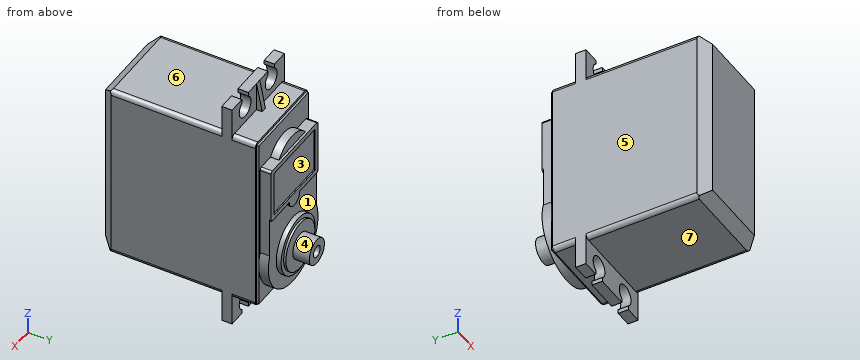
from build123d import *

# Parameters (mm, degrees)
SKETCH1_W           = 20
SKETCH1_H           = 40.5
BOSS_EXTRUDE1_DEPTH = 35.2
CHAMFER1_SIZE       = 2
CHAMFER1_SIZE2      = 2.383507185
BOSS_EXTRUDE2_DEPTH = 2.3
SKETCH3_W           = 1.25
SKETCH3_H           = 6.5
BOSS_EXTRUDE3_DEPTH = 1.3
CHAMFER2_SIZE       = 6.687920221
CHAMFER2_SIZE_2     = 1.3
SKETCH5_OUTSIDE_W   = 35.418
SKETCH5_OUTSIDE_H   = 68.918
SKETCH5_OUTSIDE_W_2 = 19
SKETCH5_OUTSIDE_H_2 = 39.5
CUT_EXTRUDE1_DEPTH  = 0.5
BOSS_EXTRUDE4_DEPTH = 2.15
BOSS_EXTRUDE5_DEPTH = 1.9
SKETCH8_R           = 6.5
BOSS_EXTRUDE6_DEPTH = 1.1
SKETCH9_R           = 5.55
BOSS_EXTRUDE7_DEPTH = 0.5
SKETCH10_R          = 2.9
SKETCH10_R_2        = 1.3
BOSS_EXTRUDE8_DEPTH = 3.7
SKETCH11_W          = 15.8
SKETCH11_H          = 10.3
BOSS_EXTRUDE9_DEPTH = 0.3
FILLET1_R           = 0.5
FILLET2_R           = 1


with BuildPart() as part:
    # Sketch1 → Boss-Extrude1 (new body)
    with BuildSketch(Plane(origin=(0, 0, 0), x_dir=(1, 0, 0), z_dir=(0, 1, 0))):
        with Locations((0, -10.25)):
            Rectangle(SKETCH1_W, SKETCH1_H)
    extrude(amount=BOSS_EXTRUDE1_DEPTH)

    # Chamfer1
    chamfer1_edges = [part.edges().sort_by_distance(p)[0] for p in [
        (0, 0, 30.5),
        (-10, 0, 10.25),
        (0, 0, -10),
        (10, 0, 10.25),
    ]]
    chamfer1_side = [part.faces().sort_by_distance(p)[0] for p in [
        (0, 0, 10.25),
    ]]
    chamfer(chamfer1_edges, length=CHAMFER1_SIZE, length2=CHAMFER1_SIZE2, reference=chamfer1_side[0])

    # Sketch2 → Boss-Extrude2 (add)
    with BuildSketch(Plane(origin=(0, 27.2, 0), x_dir=(-1, 0, 0), z_dir=(0, 1, 0))):
        with BuildLine():
            Line((10, -10), (-10, -10))
            Line((-10, -10), (-10, -16.5))
            Line((-10, -16.5), (-6.25, -16.5))
            Line((-6.25, -16.5), (-6.25, -15.570828693))
            ThreePointArc((-6.25, -15.570828693), (-5, -11.45), (-3.75, -15.570828693))
            Line((-3.75, -15.570828693), (-3.75, -16.5))
            Line((-3.75, -16.5), (3.75, -16.5))
            Line((3.75, -16.5), (3.75, -15.570828693))
            ThreePointArc((3.75, -15.570828693), (5, -11.45), (6.25, -15.570828693))
            Line((6.25, -15.570828693), (6.25, -16.5))
            Line((6.25, -16.5), (10, -16.5))
            Line((10, -16.5), (10, -10))
        make_face()
        with BuildLine():
            Line((-6.25, 37), (-10, 37))
            Line((-10, 37), (-10, 30.5))
            Line((-10, 30.5), (10, 30.5))
            Line((10, 30.5), (10, 37))
            Line((10, 37), (6.25, 37))
            Line((6.25, 37), (6.25, 36.070828693))
            ThreePointArc((6.25, 36.070828693), (5, 31.95), (3.75, 36.070828693))
            Line((3.75, 36.070828693), (3.75, 37))
            Line((3.75, 37), (-3.75, 37))
            Line((-3.75, 37), (-3.75, 36.070828693))
            ThreePointArc((-3.75, 36.070828693), (-5, 31.95), (-6.25, 36.070828693))
            Line((-6.25, 36.070828693), (-6.25, 37))
        make_face()
    extrude(amount=BOSS_EXTRUDE2_DEPTH)

    # Sketch3 → Boss-Extrude3 (add)
    with BuildSketch(Plane(origin=(0, 29.5, 0), x_dir=(1, 0, 0), z_dir=(0, 1, 0))):
        with Locations((0, -33.75)):
            Rectangle(SKETCH3_W, SKETCH3_H)
        with Locations((0, 13.25)):
            Rectangle(SKETCH3_W, SKETCH3_H)
    extrude(amount=BOSS_EXTRUDE3_DEPTH)

    # Chamfer2
    # the kernel refuses this chamfer: 6.687920221, 1.3 mm, written as the material it takes off along each edge
    with BuildSketch(Plane(origin=(-18.001773564, 30.8, 37), x_dir=(0, 0.007343799087842576, -0.9999730339438946), z_dir=(1, 0, 0))) as chamfer2_piece_1_section:
        Polygon((CHAMFER2_SIZE * 0.999973033908, -CHAMFER2_SIZE * 0.00734379908758), (-CHAMFER2_SIZE_2 * 0.00734379908784, -CHAMFER2_SIZE_2 * 0.999973033944), (0, 0), align=None)
    chamfer2_piece_1 = extrude(amount=36.003547128, mode=Mode.PRIVATE)
    chamfer2_piece_1 = split(chamfer2_piece_1, bisect_by=Plane(origin=(0, 30.433956973, 30.5), z_dir=(0, 0, 1)), keep=Keep.TOP, mode=Mode.PRIVATE)
    add(chamfer2_piece_1, mode=Mode.SUBTRACT)
    with BuildSketch(Plane(origin=(18.001773564, 30.8, -16.5), x_dir=(0, -0.9816291836389949, -0.19079870499623547), z_dir=(-1, 0, 0))) as chamfer2_piece_2_section:
        Polygon((CHAMFER2_SIZE_2 * 0.981629183639, CHAMFER2_SIZE_2 * 0.190798704996), (-CHAMFER2_SIZE * 0.190798704989, CHAMFER2_SIZE * 0.981629183604), (0, 0), align=None)
    chamfer2_piece_2 = extrude(amount=36.003547128, mode=Mode.PRIVATE)
    chamfer2_piece_2 = split(chamfer2_piece_2, bisect_by=Plane(origin=(0, 30.433956973, -10), z_dir=(0, 0, -1)), keep=Keep.TOP, mode=Mode.PRIVATE)
    add(chamfer2_piece_2, mode=Mode.SUBTRACT)

    # Sketch5 outside → Cut-Extrude1 (cut)
    with BuildSketch(Plane(origin=(0, 35.2, 0), x_dir=(1, 0, 0), z_dir=(0, 1, 0))):
        with Locations((0, -10.25)):
            Rectangle(SKETCH5_OUTSIDE_W, SKETCH5_OUTSIDE_H)
        with Locations((0, -10.25)):
            Rectangle(SKETCH5_OUTSIDE_W_2, SKETCH5_OUTSIDE_H_2, mode=Mode.SUBTRACT)
    extrude(amount=-CUT_EXTRUDE1_DEPTH, mode=Mode.SUBTRACT)

    # Sketch6 → Boss-Extrude4 (add)
    with BuildSketch(Plane(origin=(0, 35.2, 0), x_dir=(1, 0, 0), z_dir=(0, 1, 0))):
        with BuildLine():
            Line((-9, -3.041381265), (-9, -24.1))
            Line((-9, -24.1), (9, -24.1))
            Line((9, -24.1), (9, -3.041381265))
            ThreePointArc((9, -3.041381265), (0, 9.5), (-9, -3.041381265))
        make_face()
    extrude(amount=BOSS_EXTRUDE4_DEPTH)

    # Sketch7 → Boss-Extrude5 (add)
    with BuildSketch(Plane(origin=(0, 35.2, 0), x_dir=(1, 0, 0), z_dir=(0, 1, 0))):
        with BuildLine():
            Line((-5, -24.1), (5, -24.1))
            ThreePointArc((5, -24.1), (0, -26.6), (-5, -24.1))
        make_face()
    extrude(amount=BOSS_EXTRUDE5_DEPTH)

    # Sketch8 → Boss-Extrude6 (add)
    with BuildSketch(Plane(origin=(0, 37.35, 0), x_dir=(1, 0, 0), z_dir=(0, 1, 0))):
        with Locations(Location((0, 0, 0), (0, 0, 270))):
            Circle(SKETCH8_R)
    extrude(amount=BOSS_EXTRUDE6_DEPTH)

    # Sketch9 → Boss-Extrude7 (add)
    with BuildSketch(Plane(origin=(0, 38.45, 0), x_dir=(1, 0, 0), z_dir=(0, 1, 0))):
        with Locations(Location((0, 0, 0), (0, 0, 270))):
            Circle(SKETCH9_R)
    extrude(amount=BOSS_EXTRUDE7_DEPTH)

    # Sketch10 → Boss-Extrude8 (add)
    with BuildSketch(Plane(origin=(0, 38.95, 0), x_dir=(1, 0, 0), z_dir=(0, 1, 0))):
        with Locations(Location((0, 0, 0), (0, 0, 270))):
            Circle(SKETCH10_R)
        with Locations(Location((0, 0, 0), (0, 0, 270))):
            Circle(SKETCH10_R_2, mode=Mode.SUBTRACT)
    extrude(amount=BOSS_EXTRUDE8_DEPTH)

    # Sketch11 → Boss-Extrude9 (add)
    with BuildSketch(Plane(origin=(0, 37.35, 0), x_dir=(1, 0, 0), z_dir=(0, 1, 0))):
        with BuildLine():
            Line((-9, -24.1), (9, -24.1))
            Line((9, -24.1), (9, -11.6))
            Line((9, -11.6), (2, -11.6))
            ThreePointArc((2, -11.6), (0, -9.6), (-2, -11.6))
            Line((-2, -11.6), (-9, -11.6))
            Line((-9, -11.6), (-9, -24.1))
        make_face()
        with Locations((0, -17.85)):
            Rectangle(SKETCH11_W, SKETCH11_H, mode=Mode.SUBTRACT)
    extrude(amount=BOSS_EXTRUDE9_DEPTH)

    # Fillet1
    fillet1_edges = [part.edges().sort_by_distance(p)[0] for p in [
        (-9, 36.425, 24.1),
        (9, 36.425, 24.1),
        (-9, 37.5, 11.6),
        (9, 37.5, 11.6),
    ]]
    fillet(fillet1_edges, radius=FILLET1_R)

    # Fillet2
    fillet2_edges = [part.edges().sort_by_distance(p)[0] for p in [
        (10, 14.791753593, -10),
        (10, 32.1, -10),
        (10, 32.1, 30.5),
        (10, 14.791753593, 30.5),
        (-10, 32.1, 30.5),
        (-10, 14.791753593, 30.5),
        (-10, 14.791753593, -10),
        (-10, 32.1, -10),
    ]]
    fillet(fillet2_edges, radius=FILLET2_R)


solid = part.part
Read the model definition and answer for the solid it produces. Units are mm, in the model's axes. Face numbers are marked on the shaded views. A direction names the side the tool comes from. Give positions to 0.01 mm unless a question says otherwise; leave off trailing zeros. Write each loop counter-clockwise with the first axis right and the second up, starting at its lowest first coordinate (ties: lowest second). Pieces come first, ordered by that corner, then holes. Notation, with made-up numbers: M 32.25,43.5 L 67.25,43.5 A12 cw 67.25,47.5 Z; hole C -21.75,64 d6. An arc over 180 degrees is marked long. One line per item, written item: value. Start each with the question number.
(1) Determine the mould class of the marked faces 1, 2, 3 and 4 for opening direction Z: pulls with the +Z half, pulls with the -Z half, needs draft (parallel to the pull), parting line crosses it, or undercut.
(2) Find the intervals of material crossed by line 1 (X direction, y = 27.85, z = -13.7); line 2 (X direction, y = 41.6, z = 0); line 3 (Y direction, x = -7.75, z = 20), in increasing order.
(3) A tool of negligible diameter and unlimited length cuts with its end or side. For the marked faces 5, 6 and 7, from which of +Z, -Z, +X, -X, +Y, -Y can it reach the whole face along a straight path? Write none if from no direction.
(4) Find section A-A (y = 3). Determine the outline of the cut face in (x, z).
(5) Find section B-B (z = -13.7). Determine the outline of the cut face in (x, y) (3 decimals).
(6) Flat-ended cylindrical pins translate along their axes: pin 1 Ø4 at (x, y) = (-1, 15.5) entering from +Z; pin 2 Ø2.5 at (y, z) = (36.5, 18) entering from +X; pin 3 Ø6 at (x, y) = (-0.5, 18.5) entering from -Z. Find the tip coordinate at first contact, or state that the pin passes through.
Results below:
1. face 1: undercut
1. face 2: pulls with the +Z half
1. face 3: undercut
1. face 4: parting line crosses it
2. line 1: x = -10 to -7.25, -2.75 to 2.75, 7.25 to 10
2. line 2: x = -2.9 to -1.3, 1.3 to 2.9
2. line 3: y = 0 to 37.35
3. face 5: +Z, -Z, -X, +Y, -Y
3. face 6: +Z, +X, -X, -Y
3. face 7: -Z, +X, -X, -Y
4. outline: M -10,-9 A1 ccw -9,-10 L 9,-10 A1 ccw 10,-9 L 10,29.5 A1 ccw 9,30.5 L -9,30.5 A1 ccw -10,29.5 Z
5. outline: M -10,27.2 L -7.25,27.2 L -7.25,29.5 L -10,29.5 Z; M -2.75,27.2 L 2.75,27.2 L 2.75,29.5 L 0.625,29.5 L 0.625,30.044 L -0.625,30.044 L -0.625,29.5 L -2.75,29.5 Z; M 7.25,27.2 L 10,27.2 L 10,29.5 L 7.25,29.5 Z
6. pin 1: stops at z = 30.5
6. pin 2: stops at x = 9
6. pin 3: stops at z = -10
